Part print with two shaded views. Sizes in mm from the minimum x, y, z corner. Round coordinates to 2 decimals unless told otherwise and drop trailing zeros. Write each loop counter-clockwise with the first axis right and the second up, starting at its lowest first coordinate (ties: lowest second). Pieces come first, ordered by that corner, then holes. Notation, with made-up numbers: (54, 88) -> (81, 88) arc R14 ccw to (81, 103) -> close; hole circle Ø1 at (-19.75, 53). An arc over 180 degrees is marked (long way). Answer in a Markdown table with one row per item.
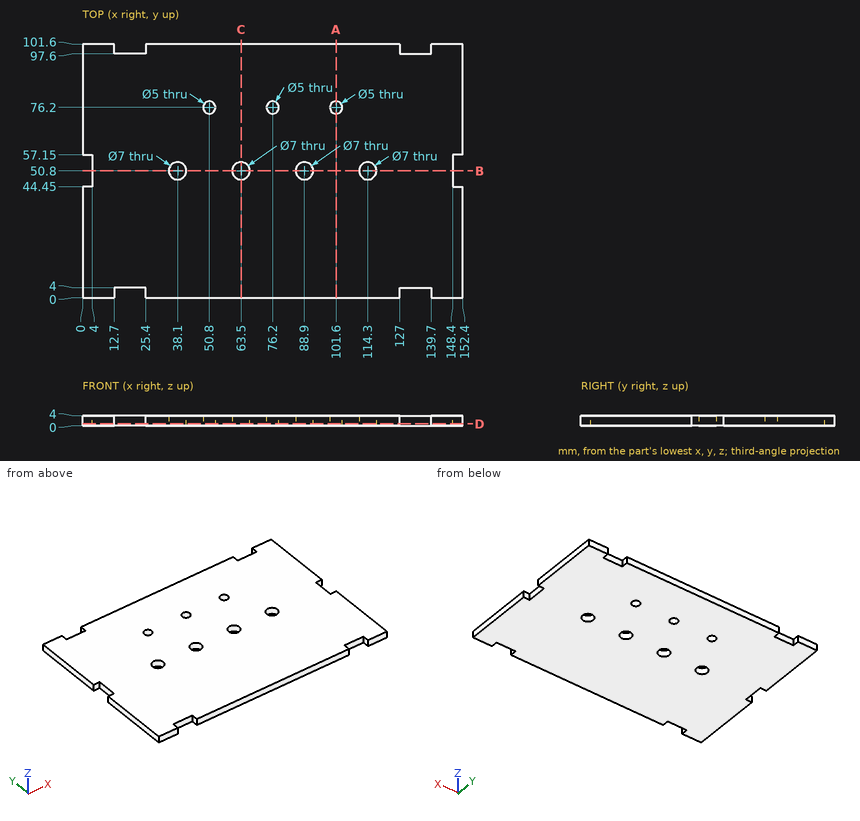
Q1. Saw through at B-B on y = 50.8. Write the cut outline in (x, z).
A:
| item | result |
|---|---|
| outline | (4, 0) -> (34.6, 0) -> (34.6, 4) -> (4, 4) -> close; (41.6, 0) -> (60, 0) -> (60, 4) -> (41.6, 4) -> close; (67, 0) -> (85.4, 0) -> (85.4, 4) -> (67, 4) -> close; (92.4, 0) -> (110.8, 0) -> (110.8, 4) -> (92.4, 4) -> close; (117.8, 0) -> (148.4, 0) -> (148.4, 4) -> (117.8, 4) -> close |
Q2. Saw through at C-C on x = 63.5. Write the cut outline in (y, z), plus the area to 3 significant figures.
A:
| item | result |
|---|---|
| outline | (0, 0) -> (47.3, 0) -> (47.3, 4) -> (0, 4) -> close; (54.3, 0) -> (101.6, 0) -> (101.6, 4) -> (54.3, 4) -> close |
| area | 378 mm² |
Q3. Saw through at D-D on z = 0.7. State how many separate pieces and enclosed holes the cut face has, plus the area to 3 significant figures.
A:
| item | result |
|---|---|
| separate pieces | 1 |
| enclosed holes | 7 |
| area | 15,000 mm² |
Q4. Saw through at A-A on x = 101.6. Write the cut outline in (y, z).
A:
| item | result |
|---|---|
| outline | (0, 0) -> (73.7, 0) -> (73.7, 4) -> (0, 4) -> close; (78.7, 0) -> (101.6, 0) -> (101.6, 4) -> (78.7, 4) -> close |
Q5. Wall check: line 1 (X direction, y = 51, z = 3.6); line 2 (Y direction, x = 101.6, z = 1.85); line 3 (Y direction, x = 38.1, z = 1.8). Give the ranges that are in metal, low to high. Write a range as [from, to].
A:
| item | result |
|---|---|
| line 1 | [4, 34.61], [41.59, 60.01], [66.99, 85.41], [92.39, 110.81], [117.79, 148.4] |
| line 2 | [0, 73.7], [78.7, 101.6] |
| line 3 | [0, 47.3], [54.3, 101.6] |
Q6. Drop flat-ended pins along their axis: P1, Ø2, axis at y = 48.5, z = 1.5, coming from the -X side; P2, Ø2, axis at x = 131.5, z = 3, coming from the +Y side; P3, Ø4, axis at x = 50.8, y = 76.2, coming from the -Z side (1 decimal). Give the stop position or say it passes through.
A:
| item | result |
|---|---|
| P1 | x = 4 |
| P2 | y = 97.6 |
| P3 | through |
